```python
from build123d import *

# Parameters (mm, degrees)
SALIENTE_EXTRUIR2_DEPTH = 228.6
REDONDEO1_R             = 2
CROQUIS3_R              = 5
CORTAR_EXTRUIR1_DEPTH   = 151
CROQUIS4_W              = 5
CROQUIS4_H              = 10
CORTAR_EXTRUIR2_DEPTH   = 10
CROQUIS5_R              = 5
CORTAR_EXTRUIR3_DEPTH   = 10


with BuildPart() as part:
    # Croquis2 → Saliente-Extruir2 (new body, symmetric)
    with BuildSketch(Plane.XY):
        Polygon((-75, 20), (-55, 20), (-55, 18), (-73, 18), (-73, -18), (73, -18), (73, 18), (55, 18), (55, 20), (75, 20), (75, -20), (-75, -20), align=None)
    extrude(amount=SALIENTE_EXTRUIR2_DEPTH, both=True)

    # Redondeo1
    redondeo1_edges = [part.edges().sort_by_distance(p)[0] for p in [
        (75, 20, 0),
        (75, -20, 0),
        (-75, -20, 0),
        (-75, 20, 0),
        (-73, 18, 0),
        (-73, -18, 0),
        (73, -18, 0),
        (73, 18, 0),
    ]]
    fillet(redondeo1_edges, radius=REDONDEO1_R)

    # Croquis3 → Cortar-Extruir1 (cut, through all)
    with BuildSketch(Plane(origin=(75, 0, 0), x_dir=(0, 0, -1), z_dir=(1, 0, 0))):
        with Locations((-211.1, 0)):
            Circle(CROQUIS3_R)
    extrude(amount=-CORTAR_EXTRUIR1_DEPTH, mode=Mode.SUBTRACT)

    # Croquis4 → Cortar-Extruir2 (cut)
    with BuildSketch(Plane(origin=(0, 20, 0), x_dir=(1, 0, 0), z_dir=(0, 1, 0))):
        with Locations((-57.5, 0.1)):
            Rectangle(CROQUIS4_W, CROQUIS4_H)
        with Locations((57.5, 0.1)):
            Rectangle(CROQUIS4_W, CROQUIS4_H)
    extrude(amount=-CORTAR_EXTRUIR2_DEPTH, mode=Mode.SUBTRACT)

    # Croquis5 → Cortar-Extruir3 (cut)
    with BuildSketch(Plane.XZ.offset(20)):
        with Locations((-37.644195885, -70)):
            Circle(CROQUIS5_R)
        with Locations((32.355804115, -70)):
            Circle(CROQUIS5_R)
        with Locations((32.355804115, 70)):
            Circle(CROQUIS5_R)
        with Locations((-37.644195885, 70)):
            Circle(CROQUIS5_R)
        with BuildLine():
            Line((-10, -208.6), (10, -208.6))
            ThreePointArc((10, -208.6), (15, -213.6), (10, -218.6))
            Line((10, -218.6), (-10, -218.6))
            ThreePointArc((-10, -218.6), (-15, -213.6), (-10, -208.6))
        make_face()
    extrude(amount=-CORTAR_EXTRUIR3_DEPTH, mode=Mode.SUBTRACT)


solid = part.part
```
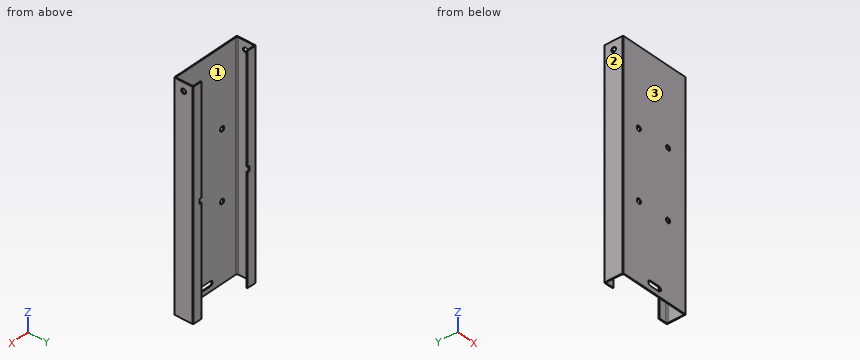
Source: CAD feature listing. Evaluate the final solid. Frame: model axes, mm. Face numbers are marked on the shaded views. Round coordinates to 2 decimals unless told otherwise and drop trailing zeros. Loops run counter-clockwise (first coordinate to the right, second up) from the corner with the lowest first, then second, coordinate; pieces in that order, holes last.
(1) Pull-direction query (Y, two-part tool) for the marked faces 1, 2 and 3; classes: +Y half, -Y half, draft (parallel to the pull), parting line (faces both ways), or undercut.
From the geometry:
face 1: undercut
face 2: draft
face 3: -Y half
(2) Contact query for flat-ended pins moving along their axis: pin 1 Ø16 at (y, z) = (0, 211.1) entering from -X; pin 2 Ø13 at (x, z) = (-37.64, -70) entering from +Y; pin 3 Ø1 at (y, z) = (19, -116.5) entering from -X; pin 4 Ø1 at (y, z) = (19.5, 118.5) entering from -X. Output: stop coordinate, or through.
From the geometry:
pin 1: stops at x = -75
pin 2: stops at y = -18
pin 3: stops at x = -74.94
pin 4: stops at x = -74.73
(3) Material intervals for probe 1 along X at (y, z) = (5.5, 127); probe 2 along Y at (x, z) = (-63, 85); probe 3 along Y at (x, z) = (30, 174.5), sorted ascending.
From the geometry:
probe 1: x = -75 to -73, 73 to 75
probe 2: y = -20 to -18, 18 to 20
probe 3: y = -20 to -18
(4) Section query C-C (z = -213.6). Output: boundary loops of the cut face in (x, y), and give its area (3 significant figures).
From the geometry:
outline: (-75, -18) arc R2 ccw to (-73, -20) - (-15, -20) - (-15, -18) - (-71, -18) arc R2 cw to (-73, -16) - (-73, 16) arc R2 cw to (-71, 18) - (-55, 18) - (-55, 20) - (-73, 20) arc R2 ccw to (-75, 18) - close; (15, -20) - (73, -20) arc R2 ccw to (75, -18) - (75, 18) arc R2 ccw to (73, 20) - (55, 20) - (55, 18) - (71, 18) arc R2 cw to (73, 16) - (73, -16) arc R2 cw to (71, -18) - (15, -18) - close
area: 464 mm2
(5) Section query D-D (z = 128.5). Output: boundary loops of the cut face in (x, y), and give its area (3 significant figures).
From the geometry:
outline: (-75, -18) arc R2 ccw to (-73, -20) - (73, -20) arc R2 ccw to (75, -18) - (75, 18) arc R2 ccw to (73, 20) - (55, 20) - (55, 18) - (71, 18) arc R2 cw to (73, 16) - (73, -16) arc R2 cw to (71, -18) - (-71, -18) arc R2 cw to (-73, -16) - (-73, 16) arc R2 cw to (-71, 18) - (-55, 18) - (-55, 20) - (-73, 20) arc R2 ccw to (-75, 18) - close
area: 524 mm2
(6) Section query B-B (z = 211.1). Output: boundary loops of the cut face in (x, y).
From the geometry:
outline: (-75, -18) arc R2 ccw to (-73, -20) - (73, -20) arc R2 ccw to (75, -18) - (75, -5) - (73, -5) - (73, -16) arc R2 cw to (71, -18) - (-71, -18) arc R2 cw to (-73, -16) - (-73, -5) - (-75, -5) - close; (-75, 5) - (-73, 5) - (-73, 16) arc R2 cw to (-71, 18) - (-55, 18) - (-55, 20) - (-73, 20) arc R2 ccw to (-75, 18) - close; (55, 18) - (71, 18) arc R2 cw to (73, 16) - (73, 5) - (75, 5) - (75, 18) arc R2 ccw to (73, 20) - (55, 20) - close
(7) Section query A-A (y = 0). Output: boundary loops of the cut face in (x, z), and give its area (3 significant figures).
From the geometry:
outline: (-75, -228.6) - (-73, -228.6) - (-73, 206.1) - (-75, 206.1) - close; (-75, 216.1) - (-73, 216.1) - (-73, 228.6) - (-75, 228.6) - close; (73, -228.6) - (75, -228.6) - (75, 206.1) - (73, 206.1) - close; (73, 216.1) - (75, 216.1) - (75, 228.6) - (73, 228.6) - close
area: 1,790 mm2
